The drawing under review shows one solid part. Ordinate dimensions are in mm from its lowest x, y, z. Round coordinates to 2 decimals unless told otherwise and drop trailing zeros. Write each loop counter-clockwise with the first axis right and the second up, starting at its lowest first coordinate (ties: lowest second). Pieces come first, ordered by that corner, then holes.
Item 1: Draft analysis for pull direction X (two halves, no side actions). For the marked faces 1, 2 and 3, state which applies: +X half, -X half, draft (parallel to the pull), parting line (faces both ways), or undercut.
Item 2: Add section D-D (z = 6.75). Give the boundary of the cut face in (x, y).
Item 3: Add section C-C (z = 1.75). Give the boundary of the cut face in (x, y).
Item 4: Clearance check with flat-ended pins moving along their axes: pin 1 Ø1 at (y, z) = (2, 1) entering from -X; pin 2 Ø1.5 at (y, z) = (7.5, 6.5) entering from -X; pin 3 Ø1.5 at (x, z) = (9.5, 5.5) entering from +Y; pin 4 Ø6 at (x, y) = (9, 9) entering from +Z. State where each tip first meets the part, or that it passes through.
Item 5: To check wall thickness, follow L1, parallel to Y at x = 5.5, z = 1.45; L2, parallel to Z at x = 4.5, y = 4.5; L3, parallel to X at y = 6, z = 4.5. State the ranges of each line that lie inside material, in increasing order.
Item 6: Add section A-A (x = 5.5). Give the boundary of the cut face in (y, z), plus the area to 3 significant figures.
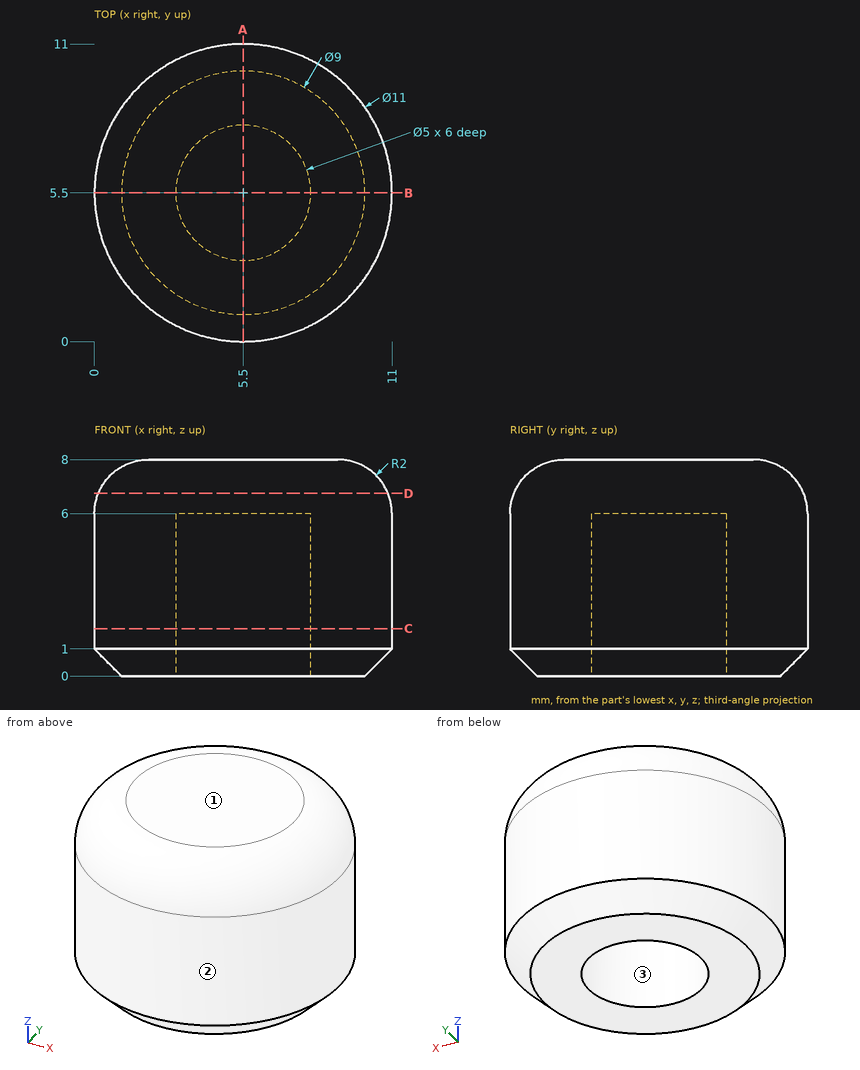
Numbers:
1. face 1: draft
1. face 2: parting line
1. face 3: undercut
2. outline: circle Ø10.71 at (5.5, 5.5)
3. outline: circle Ø11 at (5.5, 5.5); hole circle Ø5 at (5.5, 5.5)
4. pin 1: stops at x = 0.89
4. pin 2: stops at x = 0.17
4. pin 3: stops at y = 9.94
4. pin 4: stops at z = 8
5. L1: y = 0 to 3, 8 to 11
5. L2: z = 6 to 8
5. L3: x = 0.02 to 3.05, 7.95 to 10.98
6. outline: (0, 1) - (1, 0) - (3, 0) - (3, 6) - (8, 6) - (8, 0) - (10, 0) - (11, 1) - (11, 6) arc R2 ccw to (9, 8) - (2, 8) arc R2 ccw to (0, 6) - close
6. area: 55.3 mm2
